Autodesk Inventor part; units mm, degrees
ref_plane "YZ Plane" through (0, 0, 0) normal (1, 0, 0) x (0, 1, 0)
ref_plane "XZ Plane" through (0, 0, 0) normal (0, 1, 0) x (-1, 0, 0)
ref_plane "XY Plane" through (0, 0, 0) normal (0, 0, 1) x (1, 0, 0)
sketch "Sketch1" plane through (0, 0, 0) normal (0, 0, 1) x (1, 0, 0)
  line L0 (0, 0) -> (-300, 0)
  line L1 (-300, 0) -> (-550, -433.0127)
  line L2 (-550, -433.0127) -> (-550, -565.3325)
  dimension "d0" = 300
  dimension "d1" = 500
  dimension "d2" = 120
contour flange "Contour Flange1" sketch "Sketch1" thickness 5 bend radius 5 width 1000 along (0, 0, 1) mid plane yes both sides no wall seen from (-150, 0, 0) lies toward (0, 1, 0) curves L0 L1 L2
bend "Bend1"
corner "Corner1"
equation "\"d3\" = Thickness"
equation "\"d4\" = BendReliefWidth"
equation "\"d5\" = BendReliefDepth"
equation "\"d6\" = MinimumRemnant"
equation "\"d7\" = TransitionRadius"
equation "\"d9\" = BendRadius"
equation "\"d11\" = CornerReliefSize"
equation "\"d12\" = GapSize"
equation "\"d13\" = JacobiRadiusSize"
equation "\"BendRadius\" = Thickness"
equation "\"BendReliefWidth\" = Thickness"
equation "\"BendReliefDepth\" = 0.5 * Thickness"
equation "\"TransitionRadius\" = BendRadius"
equation "\"JacobiRadiusSize\" = BendRadius"
equation "\"GapSize\" = Thickness"
properties part number "Part1 example centroid" material "Copper, Wrought"
The model under review builds one solid part; all positions refer to its coordinate system, in mm. A direction names the side the tool comes from. Round coordinates to 2 decimals unless told otherwise and drop trailing zeros. Order: outer loops, then holes, each group sorted by start corner. A loop starts at its lowest first (then second) coordinate and runs counter-clockwise, first axis right, second up. Notation, with made-up numbers: (-10, -20.75) -> (39, -20.75) arc R34 ccw to (39, 10.25) -> close; hole circle Ø5 at (77.25, -33). An arc over 180 degrees is marked (long way). Use CSV: the item, a comma, the result in double quotes. Start each with the question number.
(1) Insertion check: pin 1 (6 mm diameter, centred on x = -446.5, z = 156.5, fed in from -Y); pin 2 (6 mm diameter, centred on y = -164, z = 340, fed in from +X); pin 3 (1 mm diameter, centred on y = -89, z = -158, fed in from +X). Each pin has a flat end and moves straight along its axis. Give the tip position at first contact, or say it passes through.
(2) Consider section C-C on y = -256. Write out the cut boundary in (x, z), and give its area (3 significant figures).
(3) Wall thickness on probe 1 along Y at (x, z) = (-277, -179); probe 2 along X at (y, z) = (-382, 195.5); probe 3 along X at (y, z) = (-375.5, 453.5): over which ranges is each line inside the solid? List them lowest first. Write a range as from..to.
(4) Tool access review of faces 1 (the face through (-146, 5, -7)), 2 (the face through (-550, -499, -7)): name each direction out of +Z, -Z, +X, -X, +Y, -Y from which nothing blocks a thin tool from reaching the whole face with its end or side.
(5) Consider section B-B on x = -116. Write out the cut boundary in (y, z), and give its area (3 significant figures).
(6) Consider section A-A on z = -422. Write out the cut boundary in (x, y).
Responses:
1,pin 1,"y = -258.94"
1,pin 2,"x = -392.95"
1,pin 3,"x = -351.1"
2,outline,"(-453.58, -500) -> (-447.8, -500) -> (-447.8, 500) -> (-453.58, 500) -> close"
2,area,"5,770 mm²"
3,probe 1,"0..5"
3,probe 2,"-526.32..-520.55"
3,probe 3,"-522.57..-516.8"
4,face 1,"+Z, -Z, +X, -X, +Y"
4,face 2,"+Z, -Z, +X, -Y"
5,outline,"(0, -500) -> (5, -500) -> (5, 500) -> (0, 500) -> close"
5,area,"5,000 mm²"
6,outline,"(-555, -565.33) -> (-550, -565.33) -> (-550, -434.35) arc R5 cw to (-549.33, -431.85) -> (-301.44, -2.5) arc R5 cw to (-297.11, 0) -> (0, 0) -> (0, 5) -> (-297.11, 5) arc R10 ccw to (-305.77, 0) -> (-553.66, -429.35) arc R10 ccw to (-555, -434.35) -> close"
